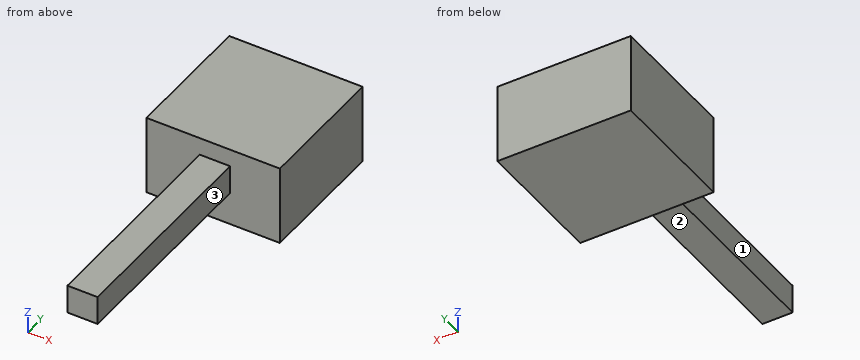
Autodesk Fusion 360 part; units mm, degrees
sketch "Sketch1" plane through (0, 0, 0) normal (0, 0, 1) x (1, 0, 0)
  line L0 (-50, 65) -> (25, 65)
  line L1 (25, 65) -> (25, -10)
  line L2 (25, -10) -> (-50, -10)
  line L3 (-50, -10) -> (-50, 65)
extrude "Extrude1" add sketch "Sketch1" along normal blind 45
sketch "Sketch2" plane through (0, -10, 0) normal (0, -1, 0) x (1, 0, 0)
  line L0 (-50, 0) -> (25, 0)
  line L1 (25, 0) -> (25, 45)
  line L2 (25, 45) -> (-50, 45)
  line L3 (-50, 45) -> (-50, 0)
  line L4 (-20, 35) -> (-2.9952, 35)
  line L5 (-2.9952, 35) -> (-2.9952, 18.7359)
  line L6 (-2.9952, 18.7359) -> (-20, 18.7359)
  line L7 (-20, 18.7359) -> (-20, 35)
extrude "Extrude2" add sketch "Sketch2" along normal blind 120 contours L4 L5 L6 L7
Can you work these out from the model? Positions are in its coordinate system, mm. Face numbers are marked on the shaded views. A direction names the side the tool comes from. Coordinates: 2 decimals unless noted, no trailing zeros. Write each loop counter-clockwise with the first axis right and the second up, starting at its lowest first coordinate (ties: lowest second). Pieces come first, ordered by that corner, then holes. Notation, with made-up numbers: M 38.25,69.25 L 86.25,69.25 A10 cw 86.25,87.25 Z; hole C 4,83 d11. An arc over 180 degrees is marked long. Answer as CSV lines item,"result".
Item 1: On a 3-axis mill with a long thin cutter (end or side, diameter ignored), from which of +Z, -Z, +X, -X, +Y, -Y can I reach the whole of each face in a straight line? I mean the marked faces 1, 2 and 3. Say none if no direction works.
Geometry results:
face 1,"+Z, -Z, -X, -Y"
face 2,"-Z, +X, -X, -Y"
face 3,"+Z, -Z, +X, -Y"
Item 2: Imagine slicing it at A-A on x = -10. List the corners of the cut face in (y, z) for me.
Geometry results:
outline,"M -130,18.74 L -10,18.74 L -10,0 L 65,0 L 65,45 L -10,45 L -10,35 L -130,35 Z"
Item 3: I'm going to push flat-ended pins straight in: P1, Ø6, axis at x = -1, z = 14.5, coming from the -Y side; P2, Ø6, axis at x = -18, y = -101.5, coming from the +Z side; P3, Ø18.5, axis at x = -10, y = -52, coming from the -Z side. Where does each tip first touch, or does it pass through?
Geometry results:
P1,"stops at y = -10"
P2,"stops at z = 35"
P3,"stops at z = 18.74"
Item 4: Imagine slicing it at D-D on x = 2. List the corners of the cut face in (y, z) for me.
Geometry results:
outline,"M -10,0 L 65,0 L 65,45 L -10,45 Z"
Item 5: Please list where these lines run through material, in increasing order: line 1 along Y through (x, z) = (-43.5, 38.5); line 2 along Z through (x, y) = (-14.5, -107); line 3 along X through (y, z) = (-13.5, 31.5).
Geometry results:
line 1,"y = -10 to 65"
line 2,"z = 18.74 to 35"
line 3,"x = -20 to -3"
Item 6: Imagine slicing it at B-B on z = 21. List the corners of the cut face in (x, y) for me, plus the area to 3 significant figures.
Geometry results:
outline,"M -50,-10 L -20,-10 L -20,-130 L -3,-130 L -3,-10 L 25,-10 L 25,65 L -50,65 Z"
area,"7,670 mm2"
Item 7: Imagine slicing it at C-C on y = -99. List the corners of the cut face in (x, z) for me, plus the area to 3 significant figures.
Geometry results:
outline,"M -20,18.74 L -3,18.74 L -3,35 L -20,35 Z"
area,"277 mm2"
